Design review of the part built by this model. Coordinates are the model's own, in mm. A direction names the side the tool comes from. Coordinates: 2 decimals unless noted, no trailing zeros. Loops run counter-clockwise (first coordinate to the right, second up) from the corner with the lowest first, then second, coordinate; pieces in that order, holes last. Notation, with made-up numbers: M -31.75,64 L -14.75,64 A25 cw -14.75,93 Z; hole C -10,68 d10. An arc over 180 degrees is marked long. Answer as a JSON object with one key per item and string values. Group by question number.
1. Consider section C-C (x = 0). State the section outline as (y, z) points, then the cut area to 3 significant figures.
2. Consider section B-B (y = 0). Count the separate pieces of the cut face and the enclosed holes in it, then the cut area to 3 significant figures.
3. Machinability: for faces 1 (the flat face through (-42.5, -45, 18)), 2 (the cylindrical face through (-29.949, 149.084, -59.984)), 3 (the cylindrical face through (-86.58, 61.03, 29.96)), which of the approach directions +Z, -Z, +X, -X, +Y, -Y give a long, thin tool a straight path to every point of the face, cutting with its end or side? Answer none if there is none.
4. Draft analysis for pull direction X (two halves, no side actions). For faces 4 (the flat face through (-87.5, -11.9, 46.4)), 5 (the cylindrical face through (-0.805, -74.927, -3.298)), 6 (the cylindrical face through (86.584, -61.491, 30.846)), state which applies: +X half, -X half, draft (parallel to the pull), parting line (faces both ways), or undercut.
5. To check wall thickness, follow probe 1 along Z at (x, y) = (85, 0); probe 2 along X at (y, z) = (-11, 79); probe 3 along X at (y, z) = (-53, -53). State the ranges of each line that lie inside material, in increasing order.
6. Insertion check: pin 1 (3 mm diameter, centred on x = -14, z = -42.5, fed in from -Y); pin 2 (12 mm diameter, centred on x = 68, y = 22, fed in from -Z); pin 3 (12 mm diameter, centred on y = -64.95, z = -37.5, fed in from -X). Each pin has a flat end and moves straight along its axis. Give the tip position at first contact, or say it passes through.
7. Consider section A-A (x = 62.5). State the section outline as (y, z) points, then the cut area to 3 significant figures.
from build123d import *

# Parameters (mm, degrees)
BOSS_EXTRUDE7_REACH      = 217.595
BOSS_EXTRUDE7_END_RADIUS = 75
SKETCH7_R                = 45
CUT_EXTRUDE1_REACH       = 284.986
SKETCH15_R               = 30
CUT_EXTRUDE2_REACH       = 261.374
SKETCH16_R               = 7.5
CUT_EXTRUDE3_REACH       = 261.374
SKETCH21_R               = 8.5
CUT_EXTRUDE4_REACH       = 284.986
SKETCH25_R               = 6


with BuildPart() as part:
    # Sketch1 → Revolve1 (revolve)
    with BuildSketch(Plane.XY, mode=Mode.PRIVATE) as revolve1_sk:
        with BuildLine():
            Line((-92.5, -95), (-92.5, -52.5))
            Line((-92.5, -52.5), (-87.5, -52.5))
            Line((-87.5, -52.5), (-87.5, -47.5))
            Line((-87.5, -47.5), (-42.5, -47.5))
            Line((-42.5, -47.5), (-42.5, -50.5))
            ThreePointArc((-42.5, -50.5), (-41.914213562, -51.914213562), (-40.5, -52.5))
            Line((-40.5, -52.5), (27.5, -52.5))
            ThreePointArc((27.5, -52.5), (28.914213562, -51.914213562), (29.5, -50.5))
            Line((29.5, -50.5), (29.5, -43.5))
            Line((29.5, -43.5), (44.5, -43.5))
            Line((44.5, -43.5), (46.5, -41.5))
            Line((46.5, -41.5), (46.5, -36))
            Line((46.5, -36), (92.5, -36))
            Line((92.5, -36), (92.5, -95))
            Line((92.5, -95), (80.5, -95))
            Line((80.5, -95), (80.5, -50))
            Line((80.5, -50), (66.5, -50))
            Line((66.5, -50), (66.5, -65))
            Line((66.5, -65), (57.5, -65))
            Line((57.5, -65), (57.5, -75))
            Line((57.5, -75), (-57.5, -75))
            Line((-57.5, -75), (-57.5, -62.5))
            Line((-57.5, -62.5), (-80.5, -62.5))
            Line((-80.5, -62.5), (-80.5, -95))
            Line((-80.5, -95), (-92.5, -95))
        make_face()
    revolve(revolve1_sk.sketch.rotate(Axis((0, 0, 0), (-1, 0, 0)), 180), axis=Axis((0, 0, 0), (-1, 0, 0)))



with BuildPart() as body_2:
    # Sketch2 → Revolve2 (revolve)
    with BuildSketch(Plane.XY, mode=Mode.PRIVATE) as revolve2_sk:
        Polygon((0, 155), (80, 155), (80, 143), (40, 143), (40, 91), (45, 91), (45, 75), (0, 75), align=None)
    revolve(revolve2_sk.sketch.rotate(Axis((0, 155, 0), (0, -1, 0)), 180), axis=Axis((0, 155, 0), (0, -1, 0)))


with BuildPart() as part_1:
    add(part.part)

    add(body_2.part)  # Boss-Extrude7 merges body 2
    # Boss-Extrude7: up to this cylinder (the profile starts outside it)
    boss_extrude7_end = Plane(origin=(0, 0, 0), z_dir=(1, 0, 0)) * Cylinder(BOSS_EXTRUDE7_END_RADIUS, 586.19, mode=Mode.PRIVATE)
    # Sketch7 → Boss-Extrude7 (add, up to the surface)
    with BuildSketch(Plane.XZ.offset(-75), mode=Mode.PRIVATE) as boss_extrude7_sk1:
        with Locations(Location((0, 0, 0), (0, 0, 180))):
            Circle(SKETCH7_R)
    boss_extrude7_tool1 = extrude(boss_extrude7_sk1.sketch, amount=BOSS_EXTRUDE7_REACH, mode=Mode.PRIVATE) - boss_extrude7_end
    add(boss_extrude7_tool1.solids().sort_by_distance((0, 75, 0))[0])
    add(boss_extrude7_tool1.solids().sort_by_distance((0, 75, 0))[1])

    # Sketch15 → Cut-Extrude1 (cut, up to next)
    with BuildSketch(Plane(origin=(0, 155, 0), x_dir=(1, 0, 0), z_dir=(0, 1, 0)), mode=Mode.PRIVATE) as cut_extrude1_sk1:
        with Locations(Location((0, 0, 0), (0, 0, 180))):
            Circle(SKETCH15_R)
    cut_extrude1_tool1 = extrude(cut_extrude1_sk1.sketch, amount=-CUT_EXTRUDE1_REACH, mode=Mode.PRIVATE) & part_1.part
    add(cut_extrude1_tool1.solids().sort_by_distance((0, 155, 0))[0], mode=Mode.SUBTRACT)

    # Sketch16 → Cut-Extrude2 (cut, up to next)
    with BuildSketch(Plane(origin=(92.5, 0, 0), x_dir=(0, 0, -1), z_dir=(1, 0, 0)), mode=Mode.PRIVATE) as cut_extrude2_sk1:
        with Locations(Location((75, 0, 0), (0, 0, 90))):
            Circle(SKETCH16_R)
    cut_extrude2_tool1 = extrude(cut_extrude2_sk1.sketch, amount=-CUT_EXTRUDE2_REACH, mode=Mode.PRIVATE) & part_1.part
    # Sketch16 → Cut-Extrude2 (cut, up to next)
    with BuildSketch(Plane(origin=(92.5, 0, 0), x_dir=(0, 0, -1), z_dir=(1, 0, 0)), mode=Mode.PRIVATE) as cut_extrude2_sk2:
        with Locations(Location((37.5, -64.951905284, 0), (0, 0, 90))):
            Circle(SKETCH16_R)
    cut_extrude2_tool2 = extrude(cut_extrude2_sk2.sketch, amount=-CUT_EXTRUDE2_REACH, mode=Mode.PRIVATE) & part_1.part
    # Sketch16 → Cut-Extrude2 (cut, up to next)
    with BuildSketch(Plane(origin=(92.5, 0, 0), x_dir=(0, 0, -1), z_dir=(1, 0, 0)), mode=Mode.PRIVATE) as cut_extrude2_sk3:
        with Locations(Location((-37.5, -64.951905284, 0), (0, 0, 90))):
            Circle(SKETCH16_R)
    cut_extrude2_tool3 = extrude(cut_extrude2_sk3.sketch, amount=-CUT_EXTRUDE2_REACH, mode=Mode.PRIVATE) & part_1.part
    # Sketch16 → Cut-Extrude2 (cut, up to next)
    with BuildSketch(Plane(origin=(92.5, 0, 0), x_dir=(0, 0, -1), z_dir=(1, 0, 0)), mode=Mode.PRIVATE) as cut_extrude2_sk4:
        with Locations(Location((-75, 0, 0), (0, 0, 90))):
            Circle(SKETCH16_R)
    cut_extrude2_tool4 = extrude(cut_extrude2_sk4.sketch, amount=-CUT_EXTRUDE2_REACH, mode=Mode.PRIVATE) & part_1.part
    # Sketch16 → Cut-Extrude2 (cut, up to next)
    with BuildSketch(Plane(origin=(92.5, 0, 0), x_dir=(0, 0, -1), z_dir=(1, 0, 0)), mode=Mode.PRIVATE) as cut_extrude2_sk5:
        with Locations(Location((-37.5, 64.951905284, 0), (0, 0, 90))):
            Circle(SKETCH16_R)
    cut_extrude2_tool5 = extrude(cut_extrude2_sk5.sketch, amount=-CUT_EXTRUDE2_REACH, mode=Mode.PRIVATE) & part_1.part
    # Sketch16 → Cut-Extrude2 (cut, up to next)
    with BuildSketch(Plane(origin=(92.5, 0, 0), x_dir=(0, 0, -1), z_dir=(1, 0, 0)), mode=Mode.PRIVATE) as cut_extrude2_sk6:
        with Locations(Location((37.5, 64.951905284, 0), (0, 0, 90))):
            Circle(SKETCH16_R)
    cut_extrude2_tool6 = extrude(cut_extrude2_sk6.sketch, amount=-CUT_EXTRUDE2_REACH, mode=Mode.PRIVATE) & part_1.part
    add(cut_extrude2_tool1.solids().sort_by_distance((92.5, 0, -75))[0], mode=Mode.SUBTRACT)
    add(cut_extrude2_tool2.solids().sort_by_distance((92.5, -64.951905, -37.5))[0], mode=Mode.SUBTRACT)
    add(cut_extrude2_tool3.solids().sort_by_distance((92.5, -64.951905, 37.5))[0], mode=Mode.SUBTRACT)
    add(cut_extrude2_tool4.solids().sort_by_distance((92.5, 0, 75))[0], mode=Mode.SUBTRACT)
    add(cut_extrude2_tool5.solids().sort_by_distance((92.5, 64.951905, 37.5))[0], mode=Mode.SUBTRACT)
    add(cut_extrude2_tool6.solids().sort_by_distance((92.5, 64.951905, -37.5))[0], mode=Mode.SUBTRACT)

    # Sketch21 → Cut-Extrude3 (cut, up to next)
    with BuildSketch(Plane.ZY.offset(92.5), mode=Mode.PRIVATE) as cut_extrude3_sk1:
        with Locations(Location((75, 0, 0), (0, 0, 270))):
            Circle(SKETCH21_R)
    cut_extrude3_tool1 = extrude(cut_extrude3_sk1.sketch, amount=-CUT_EXTRUDE3_REACH, mode=Mode.PRIVATE) & part_1.part
    # Sketch21 → Cut-Extrude3 (cut, up to next)
    with BuildSketch(Plane.ZY.offset(92.5), mode=Mode.PRIVATE) as cut_extrude3_sk2:
        with Locations(Location((37.5, -64.951905284, 0), (0, 0, 270))):
            Circle(SKETCH21_R)
    cut_extrude3_tool2 = extrude(cut_extrude3_sk2.sketch, amount=-CUT_EXTRUDE3_REACH, mode=Mode.PRIVATE) & part_1.part
    # Sketch21 → Cut-Extrude3 (cut, up to next)
    with BuildSketch(Plane.ZY.offset(92.5), mode=Mode.PRIVATE) as cut_extrude3_sk3:
        with Locations(Location((-37.5, -64.951905284, 0), (0, 0, 270))):
            Circle(SKETCH21_R)
    cut_extrude3_tool3 = extrude(cut_extrude3_sk3.sketch, amount=-CUT_EXTRUDE3_REACH, mode=Mode.PRIVATE) & part_1.part
    # Sketch21 → Cut-Extrude3 (cut, up to next)
    with BuildSketch(Plane.ZY.offset(92.5), mode=Mode.PRIVATE) as cut_extrude3_sk4:
        with Locations(Location((-75, 0, 0), (0, 0, 270))):
            Circle(SKETCH21_R)
    cut_extrude3_tool4 = extrude(cut_extrude3_sk4.sketch, amount=-CUT_EXTRUDE3_REACH, mode=Mode.PRIVATE) & part_1.part
    # Sketch21 → Cut-Extrude3 (cut, up to next)
    with BuildSketch(Plane.ZY.offset(92.5), mode=Mode.PRIVATE) as cut_extrude3_sk5:
        with Locations(Location((-37.5, 64.951905284, 0), (0, 0, 270))):
            Circle(SKETCH21_R)
    cut_extrude3_tool5 = extrude(cut_extrude3_sk5.sketch, amount=-CUT_EXTRUDE3_REACH, mode=Mode.PRIVATE) & part_1.part
    # Sketch21 → Cut-Extrude3 (cut, up to next)
    with BuildSketch(Plane.ZY.offset(92.5), mode=Mode.PRIVATE) as cut_extrude3_sk6:
        with Locations(Location((37.5, 64.951905284, 0), (0, 0, 270))):
            Circle(SKETCH21_R)
    cut_extrude3_tool6 = extrude(cut_extrude3_sk6.sketch, amount=-CUT_EXTRUDE3_REACH, mode=Mode.PRIVATE) & part_1.part
    add(cut_extrude3_tool1.solids().sort_by_distance((-92.5, 0, 75))[0], mode=Mode.SUBTRACT)
    add(cut_extrude3_tool2.solids().sort_by_distance((-92.5, -64.951905, 37.5))[0], mode=Mode.SUBTRACT)
    add(cut_extrude3_tool3.solids().sort_by_distance((-92.5, -64.951905, -37.5))[0], mode=Mode.SUBTRACT)
    add(cut_extrude3_tool4.solids().sort_by_distance((-92.5, 0, -75))[0], mode=Mode.SUBTRACT)
    add(cut_extrude3_tool5.solids().sort_by_distance((-92.5, 64.951905, -37.5))[0], mode=Mode.SUBTRACT)
    add(cut_extrude3_tool6.solids().sort_by_distance((-92.5, 64.951905, 37.5))[0], mode=Mode.SUBTRACT)

    # Sketch25 → Cut-Extrude4 (cut, up to next)
    with BuildSketch(Plane(origin=(0, 155, 0), x_dir=(1, 0, 0), z_dir=(0, 1, 0)), mode=Mode.PRIVATE) as cut_extrude4_sk1:
        with Locations(Location((62.5, 0, 0), (0, 0, 180))):
            Circle(SKETCH25_R)
    cut_extrude4_tool1 = extrude(cut_extrude4_sk1.sketch, amount=-CUT_EXTRUDE4_REACH, mode=Mode.PRIVATE) & part_1.part
    # Sketch25 → Cut-Extrude4 (cut, up to next)
    with BuildSketch(Plane(origin=(0, 155, 0), x_dir=(1, 0, 0), z_dir=(0, 1, 0)), mode=Mode.PRIVATE) as cut_extrude4_sk2:
        with Locations(Location((31.25, -54.126587737, 0), (0, 0, 180))):
            Circle(SKETCH25_R)
    cut_extrude4_tool2 = extrude(cut_extrude4_sk2.sketch, amount=-CUT_EXTRUDE4_REACH, mode=Mode.PRIVATE) & part_1.part
    # Sketch25 → Cut-Extrude4 (cut, up to next)
    with BuildSketch(Plane(origin=(0, 155, 0), x_dir=(1, 0, 0), z_dir=(0, 1, 0)), mode=Mode.PRIVATE) as cut_extrude4_sk3:
        with Locations(Location((-31.25, -54.126587737, 0), (0, 0, 180))):
            Circle(SKETCH25_R)
    cut_extrude4_tool3 = extrude(cut_extrude4_sk3.sketch, amount=-CUT_EXTRUDE4_REACH, mode=Mode.PRIVATE) & part_1.part
    # Sketch25 → Cut-Extrude4 (cut, up to next)
    with BuildSketch(Plane(origin=(0, 155, 0), x_dir=(1, 0, 0), z_dir=(0, 1, 0)), mode=Mode.PRIVATE) as cut_extrude4_sk4:
        with Locations(Location((-62.5, 0, 0), (0, 0, 180))):
            Circle(SKETCH25_R)
    cut_extrude4_tool4 = extrude(cut_extrude4_sk4.sketch, amount=-CUT_EXTRUDE4_REACH, mode=Mode.PRIVATE) & part_1.part
    # Sketch25 → Cut-Extrude4 (cut, up to next)
    with BuildSketch(Plane(origin=(0, 155, 0), x_dir=(1, 0, 0), z_dir=(0, 1, 0)), mode=Mode.PRIVATE) as cut_extrude4_sk5:
        with Locations(Location((-31.25, 54.126587737, 0), (0, 0, 180))):
            Circle(SKETCH25_R)
    cut_extrude4_tool5 = extrude(cut_extrude4_sk5.sketch, amount=-CUT_EXTRUDE4_REACH, mode=Mode.PRIVATE) & part_1.part
    # Sketch25 → Cut-Extrude4 (cut, up to next)
    with BuildSketch(Plane(origin=(0, 155, 0), x_dir=(1, 0, 0), z_dir=(0, 1, 0)), mode=Mode.PRIVATE) as cut_extrude4_sk6:
        with Locations(Location((31.25, 54.126587737, 0), (0, 0, 180))):
            Circle(SKETCH25_R)
    cut_extrude4_tool6 = extrude(cut_extrude4_sk6.sketch, amount=-CUT_EXTRUDE4_REACH, mode=Mode.PRIVATE) & part_1.part
    add(cut_extrude4_tool1.solids().sort_by_distance((62.5, 155, 0))[0], mode=Mode.SUBTRACT)
    add(cut_extrude4_tool2.solids().sort_by_distance((31.25, 155, 54.126588))[0], mode=Mode.SUBTRACT)
    add(cut_extrude4_tool3.solids().sort_by_distance((-31.25, 155, 54.126588))[0], mode=Mode.SUBTRACT)
    add(cut_extrude4_tool4.solids().sort_by_distance((-62.5, 155, 0))[0], mode=Mode.SUBTRACT)
    add(cut_extrude4_tool5.solids().sort_by_distance((-31.25, 155, -54.126588))[0], mode=Mode.SUBTRACT)
    add(cut_extrude4_tool6.solids().sort_by_distance((31.25, 155, -54.126588))[0], mode=Mode.SUBTRACT)


solid = part_1.part
Findings below:
{
 "1": {"outline": "M 43.08,-30 A52.5 cw long 43.08,30 L 155,30 L 155,80 L 143,80 L 143,40 L 91,40 L 91,45 L 60,45 A75 ccw long 60,-45 L 91,-45 L 91,-40 L 143,-40 L 143,-80 L 155,-80 L 155,-30 Z", "area": "10,600 mm^2"},
 "2": {"separate pieces": "6", "enclosed holes": "0", "area": "9,340 mm^2"},
 "3": {"face 1": "none", "face 2": "+Y", "face 3": "-X"},
 "4": {"face 4": "-X half", "face 5": "undercut", "face 6": "draft"},
 "5": {"probe 1": "z = -95 to -82.5, -67.5 to -36, 36 to 67.5, 82.5 to 95", "probe 2": "x = -92.5 to -80.5, 80.5 to 92.5", "probe 3": "x = -92.5 to -80.5, -57.5 to 57.5, 80.5 to 92.5"},
 "6": {"pin 1": "stops at y = -62.8", "pin 2": "stops at z = -62.95", "pin 3": "stops at x = -57.5"},
 "7": {"outline": "C 0,0 d130; M 143,-49.94 L 155,-49.94 L 155,-6 L 143,-6 Z; M 143,6 L 155,6 L 155,49.94 L 143,49.94 Z; hole C 0,0 d72", "area": "10,300 mm^2"}
}
